Check sheet for the modelled part. Datum: model origin and axes. Units: mm. A direction names the side the tool comes from. Coordinates: 2 decimals unless noted, no trailing zeros. Write each loop counter-clockwise with the first axis right and the second up, starting at its lowest first coordinate (ties: lowest second). Pieces come first, ordered by that corner, then holes. Notation, with made-up numbers: M 11.5,55.25 L 69.5,55.25 A13 ccw 69.5,65.25 Z; hole C -13.5,53.25 d6. An arc over 180 degrees is marked long. Answer as CSV lines item,"result".
from build123d import *

# Parameters (mm, degrees)
SKETCH_1_W                = 35
SKETCH_1_H                = 40
EXTRUDE_1_DEPTH           = 1
SKETCH_2_R                = 2.75
EXTRUDE_2_DEPTH           = 2.5
SKETCH_3_R                = 1.85
CUT_EXTRUDE_1_DEPTH       = 2.5
SKETCH_4_R                = 1.1
CUT_EXTRUDE_2_DEPTH       = 2
FILLET_1_R                = 1.265
MIRROR_9_COPY_1_SKETCH_R  = 2.75
MIRROR_9_COPY_1_DEPTH     = 2.5
MIRROR_11_COPY_1_SKETCH_R = 1.1
MIRROR_11_COPY_1_DEPTH    = 2
MIRROR_13_COPY_1_SKETCH_R = 1.85
MIRROR_13_COPY_1_DEPTH    = 2.5
SKETCH_5_W                = 26
SKETCH_5_H                = 16
CUT_EXTRUDE_3_DEPTH       = 5
EXTRUDE_16_DEPTH          = 0.5
SKETCH_11_W               = 26
SKETCH_11_H               = 16
CUT_EXTRUDE_4_DEPTH       = 5
CUT_EXTRUDE_5_DEPTH       = 5


with BuildPart() as part:
    # 草图1 → 凸台-拉伸1 (new body)
    with BuildSketch(Plane.XY):
        Rectangle(SKETCH_1_W, SKETCH_1_H)
    extrude(amount=EXTRUDE_1_DEPTH)

    # 草图2 → 凸台-拉伸2 (add)
    with BuildSketch(Plane(origin=(0, 0, 0), x_dir=(-1, 0, 0), z_dir=(0, 0, -1))):
        with Locations((-14.7, 17.2)):
            Circle(SKETCH_2_R)
    extrude_2 = extrude(amount=EXTRUDE_2_DEPTH)

    # 草图3 → 切除-拉伸1 (cut)
    with BuildSketch(Plane.XY.offset(1)):
        with Locations((14.7, 17.2)):
            Circle(SKETCH_3_R)
    cut_extrude_1 = extrude(amount=-CUT_EXTRUDE_1_DEPTH, mode=Mode.SUBTRACT)

    # 草图4 → 切除-拉伸2 (cut, symmetric)
    with BuildSketch(Plane(origin=(0, 0, -2.5), x_dir=(-1, 0, 0), z_dir=(0, 0, -1))):
        with Locations((-14.7, 17.2)):
            Circle(SKETCH_4_R)
    cut_extrude_2 = extrude(amount=CUT_EXTRUDE_2_DEPTH, both=True, mode=Mode.SUBTRACT)

    # 圆角1
    fillet_1_edges = [part.edges().sort_by_distance(p)[0] for p in [
        (-17.5, 20, 0.5),
        (17.5, 20, 0.5),
        (17.5, -20, 0.5),
        (-17.5, -20, 0.5),
    ]]
    fillet(fillet_1_edges, radius=FILLET_1_R)

    # 镜向8: 凸台-拉伸2 across plane
    add(extrude_2.mirror(Plane(origin=(0, 0, 0), x_dir=(0, 0, 1), z_dir=(1, 0, 0))))

    # 镜向9: 凸台-拉伸2 across plane
    add(extrude_2.mirror(Plane.ZX))

    # 镜向9 copy 1 sketch → 镜向9 copy 1 (add)
    with BuildSketch(Plane(origin=(0, 0, 0), x_dir=(1, 0, 0), z_dir=(0, 0, -1))):
        with Locations((-14.7, 17.2)):
            Circle(MIRROR_9_COPY_1_SKETCH_R)
    extrude(amount=MIRROR_9_COPY_1_DEPTH)

    # 镜向10: 切除-拉伸2 across plane
    add(cut_extrude_2.mirror(Plane.ZX), mode=Mode.SUBTRACT)

    # 镜向11: 切除-拉伸2 across plane
    add(cut_extrude_2.mirror(Plane(origin=(0, 0, 0), x_dir=(0, 0, 1), z_dir=(1, 0, 0))), mode=Mode.SUBTRACT)

    # 镜向11 copy 1 sketch → 镜向11 copy 1 (cut, symmetric)
    with BuildSketch(Plane(origin=(0, 0, -2.5), x_dir=(1, 0, 0), z_dir=(0, 0, -1))):
        with Locations((-14.7, 17.2)):
            Circle(MIRROR_11_COPY_1_SKETCH_R)
    extrude(amount=MIRROR_11_COPY_1_DEPTH, both=True, mode=Mode.SUBTRACT)

    # 镜向12: 切除-拉伸1 across plane
    add(cut_extrude_1.mirror(Plane(origin=(0, 0, 0), x_dir=(0, 0, 1), z_dir=(1, 0, 0))), mode=Mode.SUBTRACT)

    # 镜向13: 切除-拉伸1 across plane
    add(cut_extrude_1.mirror(Plane.ZX), mode=Mode.SUBTRACT)

    # 镜向13 copy 1 sketch → 镜向13 copy 1 (cut)
    with BuildSketch(Plane(origin=(0, 0, 1), x_dir=(-1, 0, 0), z_dir=(0, 0, 1))):
        with Locations((14.7, 17.2)):
            Circle(MIRROR_13_COPY_1_SKETCH_R)
    extrude(amount=-MIRROR_13_COPY_1_DEPTH, mode=Mode.SUBTRACT)

    # 草图5 → 切除-拉伸3 (cut, symmetric)
    with BuildSketch(Plane.XY.offset(1)):
        Rectangle(SKETCH_5_W, SKETCH_5_H)
    extrude(amount=CUT_EXTRUDE_3_DEPTH, both=True, mode=Mode.SUBTRACT)

    # 草图10 → 凸台-拉伸16 (add)
    with BuildSketch(Plane.XY.offset(1)):
        Polygon((0, 20.207259422), (-17.5, 10.103629711), (-17.5, -10.103629711), (0, -20.207259422), (17.5, -10.103629711), (17.5, 10.103629711), align=None)
    extrude(amount=EXTRUDE_16_DEPTH)

    # 草图11 → 切除-拉伸4 (cut)
    with BuildSketch(Plane(origin=(0, 0, 1), x_dir=(-1, 0, 0), z_dir=(0, 0, -1))):
        Rectangle(SKETCH_11_W, SKETCH_11_H)
    extrude(amount=-CUT_EXTRUDE_4_DEPTH, mode=Mode.SUBTRACT)

    # 草图12 → 切除-拉伸5 (cut)
    with BuildSketch(Plane(origin=(0, 0, 1), x_dir=(-1, 0, 0), z_dir=(0, 0, -1))):
        Polygon((-0.358983849, 20), (0.358983849, 20), (0, 20.207259422), align=None)
    cut_extrude_5 = extrude(amount=-CUT_EXTRUDE_5_DEPTH, mode=Mode.SUBTRACT)

    # 镜向15: 切除-拉伸5 across plane
    add(cut_extrude_5.mirror(Plane.ZX), mode=Mode.SUBTRACT)


solid = part.part
1) Mould release check, pull along X, two halves, no side actions. Record for faces 1 (the face through (13, 0, 1)), 2 (the face through (-17.14, 19.62, 0.51)), 3 (the face through (0, 20, 1)): pulls with the +X half, pulls with the -X half, needs draft (parallel to the pull), parting line crosses it, or undercut.
Answer key:
face 1,"undercut"
face 2,"pulls with the -X half"
face 3,"needs draft"
2) Depth check by flat-ended pin: P1, Ø4, axis at x = -14, y = -17.5, coming from the +Z side; P2, Ø10, axis at x = -12.5, y = 8, coming from the -Z side; P3, Ø1.9, axis at x = 15, y = 16.5, coming from the +Z side. Enter the tip coordinate at first touch or a pass-through.
Answer key:
P1,"stops at z = 1"
P2,"stops at z = 0"
P3,"stops at z = -1.5"
3) Tool access check on faces 4 (the face through (0, 9, 0)), 5 (the face through (14.299, -15.394, -0.232)), 6 (the face through (11, 17, 1)). Record the directions out of +Z, -Z, +X, -X, +Y, -Y that give a thin tool (end or side, any length) a straight path to the whole face; none if there is none.
Answer key:
face 4,"-Z"
face 5,"+Z"
face 6,"+Z, +X, +Y"
4) Section check C-C, the plane x = 8. Record the boundary of the cut face in (y, z), plus the area to 3 significant figures.
Answer key:
outline,"M -20,0 L -8,0 L -8,1.5 L -15.59,1.5 L -15.59,1 L -20,1 Z; M 8,0 L 20,0 L 20,1 L 15.59,1 L 15.59,1.5 L 8,1.5 Z"
area,"31.6 mm2"
5) Section check B-B, the plane y = -6.5. Record the boundary of the cut face in (x, z), plus the area to 3 significant figures.
Answer key:
outline,"M -17.5,0 L -13,0 L -13,1.5 L -17.5,1.5 Z; M 13,0 L 17.5,0 L 17.5,1.5 L 13,1.5 Z"
area,"13.5 mm2"
6) Section check D-D, the plane x = 14.7. Give the number of separate pieces and of enclosed holes in the cut face, plus the area to 3 significant figures.
Answer key:
separate pieces,"3"
enclosed holes,"0"
area,"56.3 mm2"
7) Section check A-A, the plane z = -1.95. Record the boundary of the cut face in (x, y).
Answer key:
outline,"C -14.7,-17.2 d5.5; C -14.7,17.2 d5.5; C 14.7,-17.2 d5.5; C 14.7,17.2 d5.5; hole C -14.7,-17.2 d2.2; hole C -14.7,17.2 d2.2; hole C 14.7,-17.2 d2.2; hole C 14.7,17.2 d2.2"
8) Thickness scan on line 1 along Y through (x, z) = (14.7, -1.75); line 2 along X through (y, z) = (-0.5, 0.15); line 3 along Y through (x, z) = (-4.5, 0.8). Record the ranges inside material, lowest first.
Answer key:
line 1,"y = -19.95 to -18.3, -16.1 to -14.45, 14.45 to 16.1, 18.3 to 19.95"
line 2,"x = -17.5 to -13, 13 to 17.5"
line 3,"y = -20 to -8, 8 to 20"
